Source: CAD feature listing. Evaluate the final solid. Frame: model axes, mm. A direction names the side the tool comes from. Round coordinates to 2 decimals unless told otherwise and drop trailing zeros. Write each loop counter-clockwise with the first axis right and the second up, starting at its lowest first coordinate (ties: lowest second). Pieces come first, ordered by that corner, then holes. Notation, with made-up numbers: M -22,34 L -12,34 A13 ccw -12,49 Z; hole C -29.5,71.25 d3. An arc over 180 degrees is marked long. Answer in a Markdown table with one row per item. Add a question column.
Item 1: Mould query, pull axis Z, two halves, no side actions, for faces 1 (the face through (10, -1, 10)), 2 (the face through (-11.52, 11.6, 19.14)), 3 (the face through (-0.54, -11.02, 7.56)). Classes: released by +Z, released by -Z, zero draft, split by the parting line, or undercut.
Item 2: Cut plane D-D on y = 3. Return loops of the section in (x, z).
Item 3: Cut plane B-B on x = -2. Return loops of the section in (y, z).
Item 4: Cut plane C-C on y = -2.5. Return loops of the section in (x, z), and give its area (3 significant figures).
Item 5: Cut plane A-A on z = 10. Return loops of the section in (x, y).
Item 6: Contact query for flat-ended pins moving along their axis: pin 1 (2 mm diameter, centred on x = -2.5, z = 16, fed in from +Y); pin 2 (7 mm diameter, centred on y = 3, z = 10, fed in from +X). Output: stop coordinate, or through.
Item 7: Material intervals for probe 1 along X at (y, z) = (-2.25, 8.75); probe 2 along Y at (x, z) = (1, 2.75); probe 3 along Z at (x, y) = (0, -10.55), sorted ascending.
Item 8: Set-up query: faces 4 (the face through (-10, -1, 10)), 5 (the face through (-11, 12.5, 10)). Return all of +Z, -Z, +X, -X, +Y, -Y with unobstructed straight access to the full face (end or side cutting, diameter ignored); none if empty.
Autodesk Inventor part; units mm, degrees
ref_plane "YZ Plane" through (0, 0, 0) normal (1, 0, 0) x (0, 1, 0)
ref_plane "XZ Plane" through (0, 0, 0) normal (0, 1, 0) x (-1, 0, 0)
ref_plane "XY Plane" through (0, 0, 0) normal (0, 0, 1) x (1, 0, 0)
sketch "Sketch1" plane through (0, 0, 0) normal (0, 0, 1) x (1, 0, 0)
  line L0 (-13, -12.5) -> (13, -12.5) construction
  line L1 (13, -12.5) -> (13, 12.5) construction
  line L2 (13, 12.5) -> (-13, 12.5) construction
  line L3 (-13, 12.5) -> (-13, -12.5) construction
  line L4 (-13, -12.5) -> (13, 12.5) construction
  line L5 (13, -12.5) -> (-13, 12.5) construction
  line L6 (-10, 12.5) -> (10, 12.5) construction
  line L7 (10, 12.5) -> (10, -9.5) construction
  line L8 (10, -9.5) -> (-10, -9.5) construction
  line L9 (-10, -9.5) -> (-10, 12.5) construction
  line L10 (-10, 12.5) -> (-13, 12.5)
  line L11 (-13, 12.5) -> (-13, -12.5)
  line L12 (-13, -12.5) -> (13, -12.5)
  line L13 (13, -12.5) -> (13, 12.5)
  line L14 (13, 12.5) -> (10, 12.5)
  line L15 (10, 12.5) -> (10, -9.5)
  line L16 (10, -9.5) -> (-10, -9.5)
  line L17 (-10, -9.5) -> (-10, 12.5)
  point P0 (0, 0)
  dimension "d0" = 26
  dimension "d1" = 25
  dimension "d2" = 3
  dimension "d3" = 3
  dimension "d4" = 3
extrude "Extrusion1" add sketch "Sketch1" along normal blind 20
sketch "Sketch2" plane through (13, -12.5, 0) normal (1, 0, 0) x (0, 0, -1)
  line L0 (-20, 25) -> (-20, 0) construction
  line L1 (0, 0) -> (0, 25) construction
  line L2 (-20, 25) -> (0, 25) construction
  line L3 (0, 25) -> (0, 5) construction
  line L4 (0, 5) -> (-20, 5) construction
  line L5 (-20, 5) -> (-20, 25) construction
  line L6 (-20, 25) -> (0, 5) construction
  line L7 (-20, 5) -> (0, 25) construction
  line L8 (0, 25) -> (-20, 25) construction
  line L9 (-10, 25) -> (-10, 5) construction
  circle A0 centre (-10, 15.5) radius 3
  line L10 (0, 25) -> (0, 0)
  line L11 (-20, 0) -> (0, 0) construction
  line L12 (0, 0) -> (0, 3) construction
  line L13 (0, 3) -> (-20, 3) construction
  line L14 (-20, 3) -> (-20, 0) construction
  point P0 (0, 12.5)
  dimension "d7" = 20
  dimension "d17" = 6
  dimension "d20" = 3
  dimension "d21" = 12.5
extrude "Extrusion2" cut sketch "Sketch2" against normal blind 39
sketch "Sketch3" plane through (-13, -12.5, 0) normal (0, -1, 0) x (1, 0, 0)
  line L0 (0, 20) -> (26, 0) construction
  line L1 (0, 0) -> (26, 20) construction
  circle A0 centre (13, 10) radius 2.5
  point P0 (13, 0)
  dimension "d11" = 5
extrude "Extrusion3" cut sketch "Sketch3" against normal blind 39
fillet "Fillet2" radius 3 2 edges at (13, -12.5, 10) (-13, -12.5, 10)
fillet "Fillet3" radius 3 4 edges at (-11.5, 12.5, 20) (-11.5, 12.5, 0) (11.5, 12.5, 20) (11.5, 12.5, 0)
equation "\"d3\" = d2"
equation "\"d4\" = d3"
properties part number "linear_actuator_connector" material "Iron, Cast"
Results below:
| question | item | result |
|---|---|---|
| 1 | face 1 | zero draft |
| 1 | face 2 | released by +Z |
| 1 | face 3 | undercut |
| 2 | outline | M -13,0 L -10,0 L -10,7 L -13,7 Z; M -13,13 L -10,13 L -10,20 L -13,20 Z; M 10,0 L 13,0 L 13,7 L 10,7 Z; M 10,13 L 13,13 L 13,20 L 10,20 Z |
| 3 | outline | M -12.5,0 L -9.5,0 L -9.5,8.5 L -12.5,8.5 Z; M -12.5,11.5 L -9.5,11.5 L -9.5,20 L -12.5,20 Z |
| 4 | outline | M -13,0 L -10,0 L -10,20 L -13,20 Z; M 10,0 L 13,0 L 13,20 L 10,20 Z |
| 4 | area | 120 mm2 |
| 5 | outline | M -13,-9.5 A3 ccw -10,-12.5 L -2.5,-12.5 L -2.5,-9.5 L -10,-9.5 L -10,0 L -13,0 Z; M -13,6 L -10,6 L -10,12.5 L -13,12.5 Z; M 2.5,-12.5 L 10,-12.5 A3 ccw 13,-9.5 L 13,0 L 10,0 L 10,-9.5 L 2.5,-9.5 Z; M 10,6 L 13,6 L 13,12.5 L 10,12.5 Z |
| 6 | pin 1 | y = -9.5 |
| 6 | pin 2 | x = 13 |
| 7 | probe 1 | -13 to -10, 10 to 13 |
| 7 | probe 2 | -12.5 to -9.5 |
| 7 | probe 3 | 0 to 7.5, 12.5 to 20 |
| 8 | face 4 | +Z, -Z, +Y |
| 8 | face 5 | +Z, -Z, +X, -X, +Y |
